```python
from build123d import *

# Parameters (mm, degrees)
SKETCH1_W                       = 13.3604
SKETCH1_H                       = 15.748
BOSS_EXTRUDE1_DEPTH             = 13.3096
CUT_EXTRUDE1_DEPTH              = 6.731
CUT_EXTRUDE2_DEPTH              = 6.4516
SKETCH4_W                       = 0.254
SKETCH4_H                       = 1.0922
CUT_EXTRUDE3_DEPTH              = 6.4516
BOSS_EXTRUDE2_REACH             = 17.835
BOSS_EXTRUDE2_DIRECTION_2_REACH = 17.835
CUT_EXTRUDE4_REACH              = 18.845
SKETCH6_W                       = 0.254
SKETCH6_H                       = 6.0452


with BuildPart() as part:
    # Sketch1 → Boss-Extrude1 (new body)
    with BuildSketch(Plane(origin=(0, 0, 0), x_dir=(1, 0, 0), z_dir=(0, 1, 0))):
        Rectangle(SKETCH1_W, SKETCH1_H)
    extrude(amount=BOSS_EXTRUDE1_DEPTH)

    # Sketch2 → Cut-Extrude1 (cut)
    with BuildSketch(Plane(origin=(0, 13.3096, 0), x_dir=(1, 0, 0), z_dir=(0, 1, 0))):
        Polygon((-2.0066, 7.3152), (-2.0066, 5.0292), (-3.2766, 5.0292), (-3.2766, 3.81), (-5.207, 3.81), (-5.207, -3.8862), (-3.2766, -3.8862), (-3.2766, -4.9784), (3.2766, -4.9784), (3.2766, -3.8862), (5.207, -3.8862), (5.207, 3.81), (3.2766, 3.81), (3.2766, 5.0292), (2.0066, 5.0292), (2.0066, 7.3152), align=None)
    extrude(amount=-CUT_EXTRUDE1_DEPTH, mode=Mode.SUBTRACT)

    # Sketch3 → Cut-Extrude2 (cut)
    with BuildSketch(Plane(origin=(0, 6.5786, 0), x_dir=(1, 0, 0), z_dir=(0, 1, 0))):
        Polygon((-3.2766, -3.8862), (3.2766, -3.8862), (5.207, -3.8862), (5.207, 3.81), (3.2766, 3.81), (3.2766, 5.0292), (2.0066, 5.0292), (2.0066, 7.3152), (-2.0066, 7.3152), (-2.0066, 5.0292), (-3.2766, 5.0292), (-3.2766, 3.81), (-5.207, 3.81), (-5.207, -3.8862), align=None)
    extrude(amount=-CUT_EXTRUDE2_DEPTH, mode=Mode.SUBTRACT)

    # Sketch4 → Cut-Extrude3 (cut)
    with BuildSketch(Plane(origin=(0, 6.5786, 0), x_dir=(1, 0, 0), z_dir=(0, 1, 0))):
        with Locations((-0.9525, -4.4323)):
            Rectangle(SKETCH4_W, SKETCH4_H)
        with Locations((-0.3175, -4.4323)):
            Rectangle(SKETCH4_W, SKETCH4_H)
        with Locations((0.3175, -4.4323)):
            Rectangle(SKETCH4_W, SKETCH4_H)
        with Locations((0.9525, -4.4323)):
            Rectangle(SKETCH4_W, SKETCH4_H)
    extrude(amount=-CUT_EXTRUDE3_DEPTH, mode=Mode.SUBTRACT)

    # Sketch5 → Boss-Extrude2 (add, up to next)
    with BuildSketch(Plane(origin=(0, 1.788865417, 0.693855168), x_dir=(-1, 0, 0), z_dir=(0, -0.9323238012155132, -0.3616245700820899)), mode=Mode.PRIVATE) as boss_extrude2_sk1:
        with BuildLine():
            Line((1.0795, -4.595554492), (0.8255, -4.595554492))
            Line((0.8255, -4.595554492), (0.8255, -2.389497415))
            ThreePointArc((0.8255, -2.389497415), (0.9525, -2.262497415), (1.0795, -2.389497415))
            Line((1.0795, -2.389497415), (1.0795, -4.595554492))
        make_face()
    boss_extrude2_tool1 = extrude(boss_extrude2_sk1.sketch, amount=BOSS_EXTRUDE2_REACH, mode=Mode.PRIVATE) - part.part
    # Sketch5 → Boss-Extrude2 (add, up to next)
    with BuildSketch(Plane(origin=(0, 1.788865417, 0.693855168), x_dir=(-1, 0, 0), z_dir=(0, -0.9323238012155132, -0.3616245700820899)), mode=Mode.PRIVATE) as boss_extrude2_sk2:
        with BuildLine():
            Line((0.4445, -4.595554492), (0.1905, -4.595554492))
            Line((0.1905, -4.595554492), (0.1905, -2.389497415))
            ThreePointArc((0.1905, -2.389497415), (0.3175, -2.262497415), (0.4445, -2.389497415))
            Line((0.4445, -2.389497415), (0.4445, -4.595554492))
        make_face()
    boss_extrude2_tool2 = extrude(boss_extrude2_sk2.sketch, amount=BOSS_EXTRUDE2_REACH, mode=Mode.PRIVATE) - part.part
    # Sketch5 → Boss-Extrude2 (add, up to next)
    with BuildSketch(Plane(origin=(0, 1.788865417, 0.693855168), x_dir=(-1, 0, 0), z_dir=(0, -0.9323238012155132, -0.3616245700820899)), mode=Mode.PRIVATE) as boss_extrude2_sk3:
        with BuildLine():
            Line((-0.1905, -4.595554492), (-0.4445, -4.595554492))
            Line((-0.4445, -4.595554492), (-0.4445, -2.389497415))
            ThreePointArc((-0.4445, -2.389497415), (-0.3175, -2.262497415), (-0.1905, -2.389497415))
            Line((-0.1905, -2.389497415), (-0.1905, -4.595554492))
        make_face()
    boss_extrude2_tool3 = extrude(boss_extrude2_sk3.sketch, amount=BOSS_EXTRUDE2_REACH, mode=Mode.PRIVATE) - part.part
    # Sketch5 → Boss-Extrude2 (add, up to next)
    with BuildSketch(Plane(origin=(0, 1.788865417, 0.693855168), x_dir=(-1, 0, 0), z_dir=(0, -0.9323238012155132, -0.3616245700820899)), mode=Mode.PRIVATE) as boss_extrude2_sk4:
        with BuildLine():
            Line((-0.8255, -4.595554492), (-1.0795, -4.595554492))
            Line((-1.0795, -4.595554492), (-1.0795, -2.389497415))
            ThreePointArc((-1.0795, -2.389497415), (-0.9525, -2.262497415), (-0.8255, -2.389497415))
            Line((-0.8255, -2.389497415), (-0.8255, -4.595554492))
        make_face()
    boss_extrude2_tool4 = extrude(boss_extrude2_sk4.sketch, amount=BOSS_EXTRUDE2_REACH, mode=Mode.PRIVATE) - part.part
    add(boss_extrude2_tool1.solids().sort_by_distance((-0.9525, 0.54398, 3.90336))[0])
    add(boss_extrude2_tool2.solids().sort_by_distance((-0.3175, 0.54398, 3.90336))[0])
    add(boss_extrude2_tool3.solids().sort_by_distance((0.3175, 0.54398, 3.90336))[0])
    add(boss_extrude2_tool4.solids().sort_by_distance((0.9525, 0.54398, 3.90336))[0])

    # Sketch5 → Boss-Extrude2 direction 2 (add, up to next)
    with BuildSketch(Plane(origin=(0, 1.788865417, 0.693855168), x_dir=(-1, 0, 0), z_dir=(0, -0.9323238012155132, -0.3616245700820899)), mode=Mode.PRIVATE) as boss_extrude2_direction_2_sk1:
        with BuildLine():
            Line((1.0795, -4.595554492), (0.8255, -4.595554492))
            Line((0.8255, -4.595554492), (0.8255, -2.389497415))
            ThreePointArc((0.8255, -2.389497415), (0.9525, -2.262497415), (1.0795, -2.389497415))
            Line((1.0795, -2.389497415), (1.0795, -4.595554492))
        make_face()
    boss_extrude2_direction_2_tool1 = extrude(boss_extrude2_direction_2_sk1.sketch, amount=-BOSS_EXTRUDE2_DIRECTION_2_REACH, mode=Mode.PRIVATE) - part.part
    # Sketch5 → Boss-Extrude2 direction 2 (add, up to next)
    with BuildSketch(Plane(origin=(0, 1.788865417, 0.693855168), x_dir=(-1, 0, 0), z_dir=(0, -0.9323238012155132, -0.3616245700820899)), mode=Mode.PRIVATE) as boss_extrude2_direction_2_sk2:
        with BuildLine():
            Line((0.4445, -4.595554492), (0.1905, -4.595554492))
            Line((0.1905, -4.595554492), (0.1905, -2.389497415))
            ThreePointArc((0.1905, -2.389497415), (0.3175, -2.262497415), (0.4445, -2.389497415))
            Line((0.4445, -2.389497415), (0.4445, -4.595554492))
        make_face()
    boss_extrude2_direction_2_tool2 = extrude(boss_extrude2_direction_2_sk2.sketch, amount=-BOSS_EXTRUDE2_DIRECTION_2_REACH, mode=Mode.PRIVATE) - part.part
    # Sketch5 → Boss-Extrude2 direction 2 (add, up to next)
    with BuildSketch(Plane(origin=(0, 1.788865417, 0.693855168), x_dir=(-1, 0, 0), z_dir=(0, -0.9323238012155132, -0.3616245700820899)), mode=Mode.PRIVATE) as boss_extrude2_direction_2_sk3:
        with BuildLine():
            Line((-0.1905, -4.595554492), (-0.4445, -4.595554492))
            Line((-0.4445, -4.595554492), (-0.4445, -2.389497415))
            ThreePointArc((-0.4445, -2.389497415), (-0.3175, -2.262497415), (-0.1905, -2.389497415))
            Line((-0.1905, -2.389497415), (-0.1905, -4.595554492))
        make_face()
    boss_extrude2_direction_2_tool3 = extrude(boss_extrude2_direction_2_sk3.sketch, amount=-BOSS_EXTRUDE2_DIRECTION_2_REACH, mode=Mode.PRIVATE) - part.part
    # Sketch5 → Boss-Extrude2 direction 2 (add, up to next)
    with BuildSketch(Plane(origin=(0, 1.788865417, 0.693855168), x_dir=(-1, 0, 0), z_dir=(0, -0.9323238012155132, -0.3616245700820899)), mode=Mode.PRIVATE) as boss_extrude2_direction_2_sk4:
        with BuildLine():
            Line((-0.8255, -4.595554492), (-1.0795, -4.595554492))
            Line((-1.0795, -4.595554492), (-1.0795, -2.389497415))
            ThreePointArc((-1.0795, -2.389497415), (-0.9525, -2.262497415), (-0.8255, -2.389497415))
            Line((-0.8255, -2.389497415), (-0.8255, -4.595554492))
        make_face()
    boss_extrude2_direction_2_tool4 = extrude(boss_extrude2_direction_2_sk4.sketch, amount=-BOSS_EXTRUDE2_DIRECTION_2_REACH, mode=Mode.PRIVATE) - part.part
    add(boss_extrude2_direction_2_tool1.solids().sort_by_distance((-0.9525, 0.54398, 3.90336))[0])
    add(boss_extrude2_direction_2_tool2.solids().sort_by_distance((-0.3175, 0.54398, 3.90336))[0])
    add(boss_extrude2_direction_2_tool3.solids().sort_by_distance((0.3175, 0.54398, 3.90336))[0])
    add(boss_extrude2_direction_2_tool4.solids().sort_by_distance((0.9525, 0.54398, 3.90336))[0])

    # Sketch6 → Cut-Extrude4 (cut, up to next)
    with BuildSketch(Plane.XZ, mode=Mode.PRIVATE) as cut_extrude4_sk1:
        with Locations((-0.9525, -0.4826)):
            Rectangle(SKETCH6_W, SKETCH6_H)
    cut_extrude4_tool1 = extrude(cut_extrude4_sk1.sketch, amount=-CUT_EXTRUDE4_REACH, mode=Mode.PRIVATE) & part.part
    # Sketch6 → Cut-Extrude4 (cut, up to next)
    with BuildSketch(Plane.XZ, mode=Mode.PRIVATE) as cut_extrude4_sk2:
        with Locations((-0.3175, -0.4826)):
            Rectangle(SKETCH6_W, SKETCH6_H)
    cut_extrude4_tool2 = extrude(cut_extrude4_sk2.sketch, amount=-CUT_EXTRUDE4_REACH, mode=Mode.PRIVATE) & part.part
    # Sketch6 → Cut-Extrude4 (cut, up to next)
    with BuildSketch(Plane.XZ, mode=Mode.PRIVATE) as cut_extrude4_sk3:
        with Locations((0.9525, -0.4826)):
            Rectangle(SKETCH6_W, SKETCH6_H)
    cut_extrude4_tool3 = extrude(cut_extrude4_sk3.sketch, amount=-CUT_EXTRUDE4_REACH, mode=Mode.PRIVATE) & part.part
    # Sketch6 → Cut-Extrude4 (cut, up to next)
    with BuildSketch(Plane.XZ, mode=Mode.PRIVATE) as cut_extrude4_sk4:
        with Locations((0.3175, -0.4826)):
            Rectangle(SKETCH6_W, SKETCH6_H)
    cut_extrude4_tool4 = extrude(cut_extrude4_sk4.sketch, amount=-CUT_EXTRUDE4_REACH, mode=Mode.PRIVATE) & part.part
    add(cut_extrude4_tool1.solids().sort_by_distance((-0.9525, 0, -0.4826))[0], mode=Mode.SUBTRACT)
    add(cut_extrude4_tool2.solids().sort_by_distance((-0.3175, 0, -0.4826))[0], mode=Mode.SUBTRACT)
    add(cut_extrude4_tool3.solids().sort_by_distance((0.9525, 0, -0.4826))[0], mode=Mode.SUBTRACT)
    add(cut_extrude4_tool4.solids().sort_by_distance((0.3175, 0, -0.4826))[0], mode=Mode.SUBTRACT)


solid = part.part
```
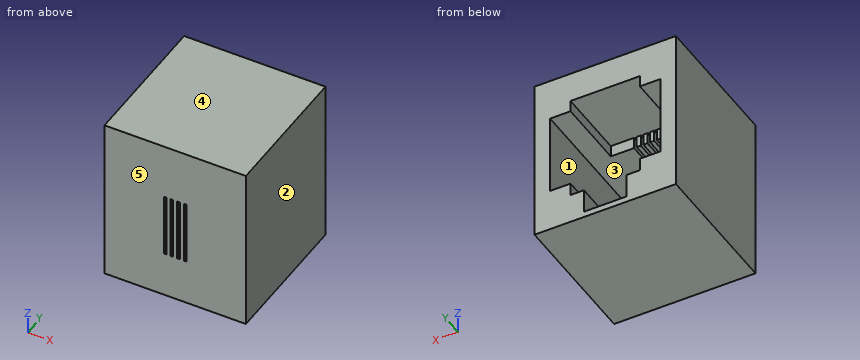
CAD build for the part. Positions are in the model's coordinates, mm. Face numbers are marked on the shaded views. A direction names the side the tool comes from. Coordinates: 2 decimals unless noted, no trailing zeros. Order: outer loops, then holes, each group sorted by start corner. A loop starts at its lowest first (then second) coordinate and runs counter-clockwise, first axis right, second up. Notation, with made-up numbers: (-26, 76) - (12, 76) arc R14 ccw to (12, 90) - close; hole circle Ø4 at (50.5, -2.5). An arc over 180 degrees is marked (long way). Use a Markdown table: item, result. Add a question column.
(1) Pull direction Z, two halves, no side cores. Call the marked faces 3, 4 and 5: +Z half, -Z half, draft (parallel to the pull), parting line (faces both ways), or undercut.
(2) Which spindle directions (+Z, -Z, +X, -X, +Y, -Y) get a long thin tool onto all of the face, cutting with end or side? Do the marked faces 1 and 2. Say none if no direction does.
(3) Saw through at D-D (z = -6). Give the cut face in (x, y).
(4) Drill centre lines: line 1 along X through (y, z) = (1, 3); line 2 along X through (y, z) = (3.5, 2.25); line 3 along Z through (x, y) = (-1.75, 8). Where is each one in solid material? Low to high. Write a range as [from, to].
(5) Saw through at C-C (x = -2.75). Give the cut face in (y, z).
(6) Saw through at A-A (z = -0.25). Give the cut face in (x, y), then the cut area to 3 significant figures.
(7) Saw through at B-B (y = 12). Give the cut face in (x, z).
Solved:
| question | item | result |
|---|---|---|
| 1 | face 3 | undercut |
| 1 | face 4 | +Z half |
| 1 | face 5 | draft |
| 2 | face 1 | +Y |
| 2 | face 2 | +Z, -Z, +X, +Y, -Y |
| 3 | outline | (-6.68, 0) - (6.68, 0) - (6.68, 13.31) - (2.01, 13.31) - (2.01, 0.13) - (-2.01, 0.13) - (-2.01, 13.31) - (-6.68, 13.31) - close |
| 4 | line 1 | x = [-6.68, -5.21], [-1.08, -0.83], [-0.44, -0.19], [0.19, 0.44], [0.83, 1.08], [5.21, 6.68] |
| 4 | line 2 | x = [-6.68, -5.21], [5.21, 6.68] |
| 4 | line 3 | z = [-7.87, -7.32], [4.98, 7.87] |
| 5 | outline | (0, -7.87) - (13.31, -7.87) - (13.31, -5.03) - (0.13, -5.03) - (0.13, 3.89) - (6.58, 3.89) - (6.58, 4.98) - (13.31, 4.98) - (13.31, 7.87) - (0, 7.87) - close |
| 6 | outline | (-6.68, 0) - (-1.08, 0) - (-1.08, 0.13) - (-5.21, 0.13) - (-5.21, 13.31) - (-6.68, 13.31) - close; (-0.83, 0) - (-0.44, 0) - (-0.44, 0.13) - (-0.83, 0.13) - close; (-0.19, 0) - (0.19, 0) - (0.19, 0.13) - (-0.19, 0.13) - close; (0.44, 0) - (0.83, 0) - (0.83, 0.13) - (0.44, 0.13) - close; (1.08, 0) - (6.68, 0) - (6.68, 13.31) - (5.21, 13.31) - (5.21, 0.13) - (1.08, 0.13) - close |
| 6 | area | 40.4 mm² |
| 7 | outline | (-6.68, -7.87) - (6.68, -7.87) - (6.68, 7.87) - (-6.68, 7.87) - close; hole (-5.21, -3.81) - (-3.28, -3.81) - (-3.28, -5.03) - (-2.01, -5.03) - (-2.01, -7.32) - (2.01, -7.32) - (2.01, -5.03) - (3.28, -5.03) - (3.28, -3.81) - (5.21, -3.81) - (5.21, 3.89) - (3.28, 3.89) - (3.28, 4.98) - (-3.28, 4.98) - (-3.28, 3.89) - (-5.21, 3.89) - close |
